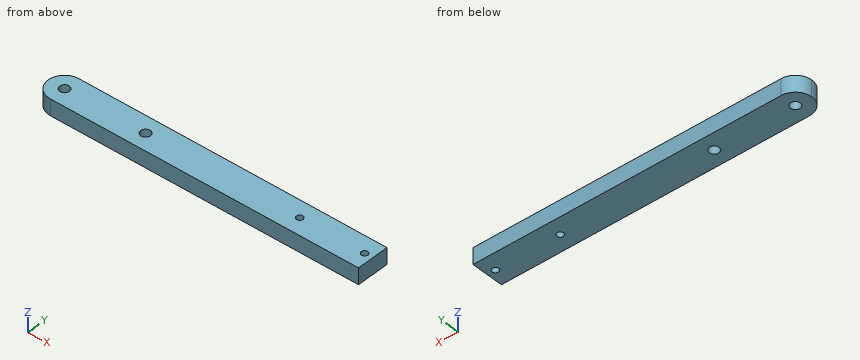
```python
from build123d import *

# Parameters (mm, degrees)
SKETCH1_W           = 200
SKETCH1_H           = 20
SKETCH1_R           = 3
SKETCH1_R_2         = 2
BOSS_EXTRUDE1_DEPTH = 10
FILLET1_R           = 10


with BuildPart() as part:
    # Sketch1 → Boss-Extrude1 (new body)
    with BuildSketch(Plane.XY):
        Rectangle(SKETCH1_W, SKETCH1_H)
        with Locations((-90, 0)):
            Circle(SKETCH1_R, mode=Mode.SUBTRACT)
        with Locations((-40, 0)):
            Circle(SKETCH1_R, mode=Mode.SUBTRACT)
        with Locations((95, 0)):
            Circle(SKETCH1_R_2, mode=Mode.SUBTRACT)
        with Locations((55, 0)):
            Circle(SKETCH1_R_2, mode=Mode.SUBTRACT)
    extrude(amount=BOSS_EXTRUDE1_DEPTH)

    # Fillet1
    fillet1_edges = [part.edges().sort_by_distance(p)[0] for p in [
        (-100, -10, 5),
        (-100, 10, 5),
    ]]
    fillet(fillet1_edges, radius=FILLET1_R - 0.0001)  # a hair under: the kernel refuses the full size


solid = part.part
```
Geometry: final body of the model. Coordinates: model frame, mm. Round coordinates to 2 decimals unless told otherwise and drop trailing zeros. Order: outer loops, then holes, each group sorted by start corner. A loop starts at its lowest first (then second) coordinate and runs counter-clockwise, first axis right, second up. Notation, with made-up numbers: M 10,77 L 60,77 A15 cw 60,82 Z; hole C -14.75,-18 d11. An arc over 180 degrees is marked long. Use one line per item in the form item = value. Start each with the question number.
Q1. Cut plane C-C (x = 55). Return loops of the section in (y, z), and give its area (3 significant figures).
Q2. Pin query (flat end, axial travel): pin 1 Ø5 at (x, y) = (-90, 0) entering from -Z; pin 2 Ø6 at (x, y) = (-39, -2.5) entering from -Z; pin 3 Ø1 at (y, z) = (7.5, 6.5) entering from -X; pin 4 Ø1.5 at (y, z) = (4, 5.5) entering from -X. Return the tip coordinate at first contact, or that it passes through.
Q3. Cut plane D-D (y = 7.75). Return loops of the section in (x, z), and give its area (3 significant figures).
Q4. Material intervals for line 1 (Y direction, x = -40, z = 3.25); line 2 (Y direction, x = 55, z = 8); line 3 (X direction, y = 0.5, z = 4.75), sorted ascending. Write a range as [from, to].
Q5. Cut plane A-A (x = -40). Return loops of the section in (y, z).
Q6. Cut plane B-B (z = 3.75). Count the separate pieces of the cut face and the enclosed holes in it, and give its area (3 significant figures).
Geometry results:
q1.outline = M -10,0 L -2,0 L -2,10 L -10,10 Z; M 2,0 L 10,0 L 10,10 L 2,10 Z
q1.area = 160 mm^2
q2.pin_1 = through
q2.pin_2 = 0
q2.pin_3 = -97.14
q2.pin_4 = -99.46
q3.outline = M -96.32,0 L 100,0 L 100,10 L -96.32,10 Z
q3.area = 1,960 mm^2
q4.line_1 = [-10, -3], [3, 10]
q4.line_2 = [-10, -2], [2, 10]
q4.line_3 = [-99.99, -92.96], [-87.04, -42.96], [-37.04, 53.06], [56.94, 93.06], [96.94, 100]
q5.outline = M -10,0 L -3,0 L -3,10 L -10,10 Z; M 3,0 L 10,0 L 10,10 L 3,10 Z
q6.separate_pieces = 1
q6.enclosed_holes = 4
q6.area = 3,880 mm^2
